Geometry: final body of the model. Coordinates: model frame, mm. Face numbers are marked on the shaded views. A direction names the side the tool comes from. Round coordinates to 2 decimals unless told otherwise and drop trailing zeros. Loops run counter-clockwise (first coordinate to the right, second up) from the corner with the lowest first, then second, coordinate; pieces in that order, holes last. Notation, with made-up numbers: (19, 88) - (60, 88) arc R27 cw to (60, 106) - close; hole circle Ø3 at (-5, 86.5). An arc over 180 degrees is marked (long way). Return JSON: item names as keys, results as strings. Group by question number.
1. Draft query along X for the marked faces 3, 4 and 5. Return one class per face: +X half, -X half, draft (parallel to the pull), parting line (faces both ways), or undercut.
2. Material intervals for probe 1 along Y at (x, z) = (0, 5.25); probe 2 along Z at (x, y) = (30, -9), sorted ascending.
3. Section C-C on z = 8.5. Return loops of the section in (x, y).
4. Section D-D on y = 24.5. Return loops of the section in (x, z) (3 decimals).
5. Set-up query: the marked faces 1 and 2. Return all of +Z, -Z, +X, -X, +Y, -Y with unobstructed straight access to the full face (end or side cutting, diameter ignored); none if empty.
6. Section A-A on x = 0. Return loops of the section in (y, z).
7. First-contact query: pin 1 Ø1 at (y, z) = (23.5, 7) entering from +X; pin 2 Ø6 at (y, z) = (-12, 4) entering from +X; pin 3 Ø1 at (y, z) = (3.5, 13) entering from -X. Flat tips, straight axial feed; report the tip coordinate or a pass-through.
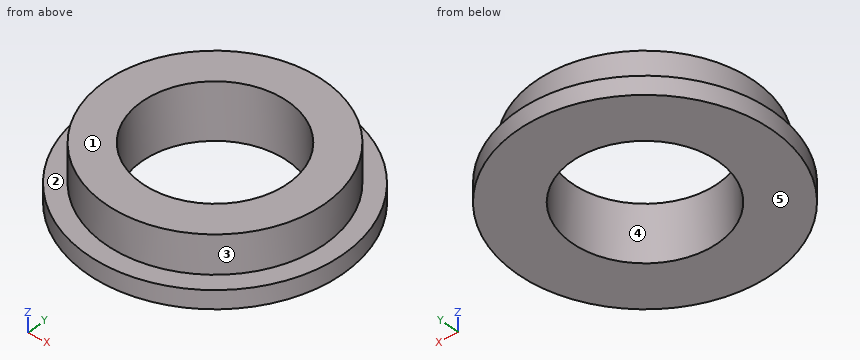
from build123d import *

# Parameters (mm, degrees)
F0_R     = 30
F1_DEPTH = 15.5
F2_R     = 35
F4_DEPTH = 5
F3_R     = 20
F5_DEPTH = 25.4
F6_D     = 40


with BuildPart() as f1:
    # F0 (on Top) → F1 (new body)
    with BuildSketch(Plane.XY):
        Circle(F0_R)
    extrude(amount=F1_DEPTH)

    # F2 (on Top) → F4 (join)
    with BuildSketch(Plane.XY):
        Circle(F2_R)
    extrude(amount=F4_DEPTH)

    # F3 (on Top) → F5 (join)
    with BuildSketch(Plane.XY):
        Circle(F3_R)
    extrude(amount=F5_DEPTH)

    # F6 (through all)
    with Locations(Plane(origin=(0, 0, 0), x_dir=(1, 0, 0), z_dir=(0, 0, -1))):
        with Locations((0, 0)):
            Hole(F6_D / 2)


solid = f1.part
Taken from the geometry:
{
 "1": {"face 3": "parting line", "face 4": "undercut", "face 5": "draft"},
 "2": {"probe 1": "-30 to -20, 20 to 30", "probe 2": "0 to 5"},
 "3": {"outline": "circle Ø60 at (0, 0); hole circle Ø40 at (0, 0)"},
 "4": {"outline": "(-24.995, 0) - (24.995, 0) - (24.995, 5) - (17.313, 5) - (17.313, 15.5) - (-17.313, 15.5) - (-17.313, 5) - (-24.995, 5) - close"},
 "5": {"face 1": "+Z, +X, -X, +Y, -Y", "face 2": "+Z"},
 "6": {"outline": "(-35, 0) - (-20, 0) - (-20, 15.5) - (-30, 15.5) - (-30, 5) - (-35, 5) - close; (20, 0) - (35, 0) - (35, 5) - (30, 5) - (30, 15.5) - (20, 15.5) - close"},
 "7": {"pin 1": "x = 19.26", "pin 2": "x = 33.82", "pin 3": "x = -29.85"}
}
